from build123d import *

# Parameters (mm, degrees)
CROQUIS1_W                 = 60
CROQUIS1_H                 = 48
SALIENTE_EXTRUIR1_DEPTH    = 6
CROQUIS4_W                 = 60
CROQUIS4_H                 = 11.5
SALIENTE_EXTRUIR3_DEPTH    = 30
CROQUIS5_R                 = 2
CORTAR_EXTRUIR3_DEPTH      = 16
CROQUIS6_W                 = 30
CROQUIS6_H                 = 48
SALIENTE_EXTRUIR4_DEPTH    = 162
CROQUIS7_R                 = 2
CORTAR_EXTRUIR4_DEPTH      = 16
CROQUIS11_W                = 150
CROQUIS11_H                = 11.5
SALIENTE_EXTRUIR6_DEPTH    = 59.25
CROQUIS12_W                = 3
CROQUIS12_H                = 150
SALIENTE_EXTRUIR7_DEPTH    = 10
CORTAR_EXTRUIR6_DEPTH      = 170.016303475
CORTAR_EXTRUIR6_DEPTH_BACK = 170.016303475
CROQUIS14_W                = 5
CROQUIS14_H                = 3.5
CORTAR_EXTRUIR7_DEPTH      = 213.768679181
CORTAR_EXTRUIR7_DEPTH_BACK = 90
CROQUIS15_W                = 11
CROQUIS15_H                = 11
CROQUIS16_W                = 30
CROQUIS16_H                = 1
CORTAR_EXTRUIR10_DEPTH     = 190.450484429
REDONDEO1_R                = 10
CROQUIS20_W                = 30
CROQUIS20_H                = 36.5
SALIENTE_EXTRUIR8_DEPTH    = 50
CROQUIS21_W                = 12
CROQUIS21_H                = 25
CORTAR_EXTRUIR11_DEPTH     = 40
CROQUIS22_W                = 30
CROQUIS22_H                = 36.5
CORTAR_EXTRUIR13_DEPTH     = 47
REDONDEO3_R                = 10


with BuildPart() as part:
    # Croquis1 → Saliente-Extruir1 (new body)
    with BuildSketch(Plane.XY):
        with Locations((-36.216216216, 7.011261261)):
            Rectangle(CROQUIS1_W, CROQUIS1_H)
    extrude(amount=SALIENTE_EXTRUIR1_DEPTH)

    # Croquis4 → Saliente-Extruir3 (add)
    with BuildSketch(Plane.XY.offset(6)):
        with Locations((-36.216216216, 25.261261261)):
            Rectangle(CROQUIS4_W, CROQUIS4_H)
        with Locations((-36.216216216, -11.238738739)):
            Rectangle(CROQUIS4_W, CROQUIS4_H)
    extrude(amount=SALIENTE_EXTRUIR3_DEPTH)

    # Croquis5 → Cortar-Extruir3 (cut)
    with BuildSketch(Plane.XY.offset(36)):
        with Locations((-51.216216216, 25.661261261)):
            Circle(CROQUIS5_R)
        with Locations((-12.216216216, 25.661261261)):
            Circle(CROQUIS5_R)
        with Locations((-12.216216216, -11.638738739)):
            Circle(CROQUIS5_R)
        with Locations((-51.216216216, -11.638738739)):
            Circle(CROQUIS5_R)
    extrude(amount=-CORTAR_EXTRUIR3_DEPTH, mode=Mode.SUBTRACT)

    # Croquis6 → Saliente-Extruir4 (add)
    with BuildSketch(Plane(origin=(0, 0, 0), x_dir=(-1, 0, 0), z_dir=(0, 0, -1))):
        with Locations((51.216216216, 7.011261261)):
            Rectangle(CROQUIS6_W, CROQUIS6_H)
    extrude(amount=SALIENTE_EXTRUIR4_DEPTH)

    # Croquis7 → Cortar-Extruir4 (cut)
    with BuildSketch(Plane(origin=(0, 0, -162), x_dir=(-1, 0, 0), z_dir=(0, 0, -1))):
        with Locations((51.216216216, 7.011261261)):
            Circle(CROQUIS7_R)
    extrude(amount=-CORTAR_EXTRUIR4_DEPTH, mode=Mode.SUBTRACT)

    # Croquis11 → Saliente-Extruir6 (add)
    with BuildSketch(Plane(origin=(-36.216216216, 0, 0), x_dir=(0, 0, -1), z_dir=(1, 0, 0))):
        with Locations((39, 25.261261261)):
            Rectangle(CROQUIS11_W, CROQUIS11_H)
    extrude(amount=SALIENTE_EXTRUIR6_DEPTH)

    # Croquis12 → Saliente-Extruir7 (add)
    with BuildSketch(Plane(origin=(0, 31.011261261, 0), x_dir=(1, 0, 0), z_dir=(0, 1, 0))):
        with Locations((14.283783784, 39)):
            Rectangle(CROQUIS12_W, CROQUIS12_H)
    extrude(amount=SALIENTE_EXTRUIR7_DEPTH)

    # Croquis14 → Cortar-Extruir6 (cut, two sides: drawn at the far end of the back side and taken through both)
    with BuildSketch(Plane(origin=(0, 0, -114), x_dir=(-1, 0, 0), z_dir=(0, 0, -1)).offset(-CORTAR_EXTRUIR6_DEPTH_BACK)):
        with Locations((-20.533783784, 21.261261261)):
            Rectangle(CROQUIS14_W, CROQUIS14_H)
    extrude(amount=CORTAR_EXTRUIR6_DEPTH + CORTAR_EXTRUIR6_DEPTH_BACK, mode=Mode.SUBTRACT)

    # Croquis15 → Cortar-Extruir7 (cut, two sides: drawn at the far end of the back side and taken through both)
    with BuildSketch(Plane(origin=(0, 0, -162), x_dir=(-1, 0, 0), z_dir=(0, 0, -1)).offset(-CORTAR_EXTRUIR7_DEPTH_BACK)):
        with Locations((51.216216216, 25.511261261)):
            Rectangle(CROQUIS15_W, CROQUIS15_H)
    extrude(amount=CORTAR_EXTRUIR7_DEPTH + CORTAR_EXTRUIR7_DEPTH_BACK, mode=Mode.SUBTRACT)

    # Croquis16 → Cortar-Extruir10 (cut, through all)
    with BuildSketch(Plane.ZY.offset(66.216216216)):
        with Locations((21, 20.011261261)):
            Rectangle(CROQUIS16_W, CROQUIS16_H)
    extrude(amount=-CORTAR_EXTRUIR10_DEPTH, mode=Mode.SUBTRACT)

    # Redondeo1
    redondeo1_edges = [part.edges().sort_by_distance(p)[0] for p in [
        (-36.216216216, -5.488738739, 6),
        (-24.091216216, 20.511261261, 6),
    ]]
    fillet(redondeo1_edges, radius=REDONDEO1_R)

    # Croquis20 → Saliente-Extruir8 (add)
    with BuildSketch(Plane(origin=(0, 0, 0), x_dir=(-1, 0, 0), z_dir=(0, 0, -1))):
        with Locations((21.216216216, 1.261261261)):
            Rectangle(CROQUIS20_W, CROQUIS20_H)
    extrude(amount=SALIENTE_EXTRUIR8_DEPTH)

    # Croquis21 → Cortar-Extruir11 (cut)
    with BuildSketch(Plane.XZ.offset(-19.511261261)):
        with Locations((-0.216216216, -0.858898944)):
            Rectangle(CROQUIS21_W, CROQUIS21_H)
        with Locations((-0.216216216, -37.5)):
            Rectangle(CROQUIS21_W, CROQUIS21_H)
    extrude(amount=-CORTAR_EXTRUIR11_DEPTH, mode=Mode.SUBTRACT)

    # Croquis22 → Cortar-Extruir13 (cut)
    with BuildSketch(Plane(origin=(0, 0, -50), x_dir=(-1, 0, 0), z_dir=(0, 0, -1))):
        with Locations((21.216216216, 1.261261261)):
            Rectangle(CROQUIS22_W, CROQUIS22_H)
    extrude(amount=-CORTAR_EXTRUIR13_DEPTH, mode=Mode.SUBTRACT)

    # Redondeo3
    redondeo3_edges = [part.edges().sort_by_distance(p)[0] for p in [
        (-21.216216216, -16.988738739, -3),
    ]]
    fillet(redondeo3_edges, radius=REDONDEO3_R)


solid = part.part
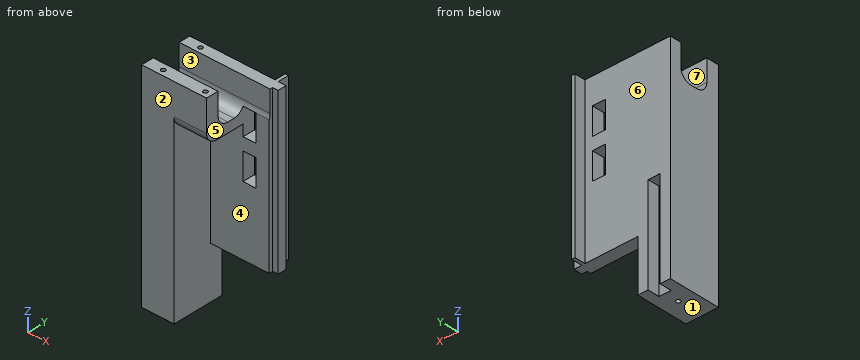
The model under review builds one solid part; all positions refer to its coordinate system, in mm. Face numbers are marked on the shaded views. A direction names the side the tool comes from. Round coordinates to 2 decimals unless told otherwise and drop trailing zeros. Loops run counter-clockwise (first coordinate to the right, second up) from the corner with the lowest first, then second, coordinate; pieces in that order, holes last. Notation, with made-up numbers: M 23.25,-6.5 L 67.25,-6.5 A22 ccw 67.25,7.5 Z; hole C 15.5,76 d4. An arc over 180 degrees is marked long. Answer as a JSON object with one key per item and string values.
Item 1: Clearance check with flat-ended pins moving along their axes: P1, Ø10, axis at y = 4.5, z = -106.5, coming from the +X side; P2, Ø23.5, axis at x = 3, y = 35, coming from the -Z side; P3, Ø4, axis at x = -23.5, z = -2.5, coming from the -Y side. State where each tip first meets the part, or that it passes through.
Check sheet entries:
{"P1": "x = -36.22", "P2": "z = -114", "P3": "y = -13.6"}
Item 2: We need section A-A, the plane x = -4. State the section outline as (y, z) points.
Check sheet entries:
{"outline": "M 19.51,-114 L 31.01,-114 L 31.01,-50 L 19.51,-50 Z; M 19.51,-25 L 31.01,-25 L 31.01,-13.36 L 19.51,-13.36 Z; M 19.51,11.64 L 31.01,11.64 L 31.01,36 L 20.51,36 L 20.51,16 A10 cw Z"}
Item 3: We need section C-C, the plane x = -30.5. State the section outline as (y, z) points.
Check sheet entries:
{"outline": "M -16.99,7 A10 ccw -6.99,-3 L 19.51,-3 L 19.51,-114 L 31.01,-114 L 31.01,36 L 20.51,36 L 20.51,16 A10 cw 10.51,6 L 4.51,6 A10 cw -5.49,16 L -5.49,36 L -16.99,36 Z"}
Item 4: We need section D-D, the plane y = -1.5. State the section outline as (x, z) points.
Check sheet entries:
{"outline": "M -66.22,-162 L -36.22,-162 L -36.22,-3 L -6.22,-3 L -6.22,8.01 L -66.22,8.01 Z"}
Item 5: Tool access review of the marked faces 4, 5, 6 and 7: name each direction out of +Z, -Z, +X, -X, +Y, -Y from which nothing blocks a thin tool from reaching the whole face with its end or side.
Check sheet entries:
{"face 4": "-Z, +X, -Y", "face 5": "-Y", "face 6": "+Z, -Z, -X, +Y", "face 7": "+Z, +X, -X"}
Item 6: We need section B-B, the plane z = -117.5. State the section outline as (x, y) points, and give its area (3 significant figures).
Check sheet entries:
{"outline": "M -66.22,-16.99 L -36.22,-16.99 L -36.22,31.01 L -45.72,31.01 L -45.72,20.01 L -56.72,20.01 L -56.72,31.01 L -66.22,31.01 Z", "area": "1,320 mm2"}
Item 7: The part is to be moulded in two halves that separate along Y. For the marked faces 1, 2 and 3, say which applies: +Y half, -Y half, draft (parallel to the pull), parting line (faces both ways), or undercut.
Check sheet entries:
{"face 1": "draft", "face 2": "-Y half", "face 3": "undercut"}
Item 8: For line 1 along Z through (x, y) = (1.5, 23.5); line 2 along Y through (x, z) = (-10.5, 18); line 3 along X through (y, z) = (-6.5, -0.5), list the stretches that pass through material, from the lowest coordinate up.
Check sheet entries:
{"line 1": "-114 to -50, -25 to -13.36, 11.64 to 36", "line 2": "-16.99 to -5.49, 20.51 to 31.01", "line 3": "-66.22 to -6.22"}
